Could you check a few things on this model? Use its own coordinates, in mm. Face numbers are marked on the shaded views. A direction names the side the tool comes from. Round coordinates to 2 decimals unless told otherwise and drop trailing zeros. Loops run counter-clockwise (first coordinate to the right, second up) from the corner with the lowest first, then second, coordinate; pieces in that order, holes last. Notation, with made-up numbers: M 19,-14.5 L 54,-14.5 A16 ccw 54,-6.5 Z; hole C 48,-10.75 d10. An arc over 180 degrees is marked long. Answer in a Markdown table with one row per item.
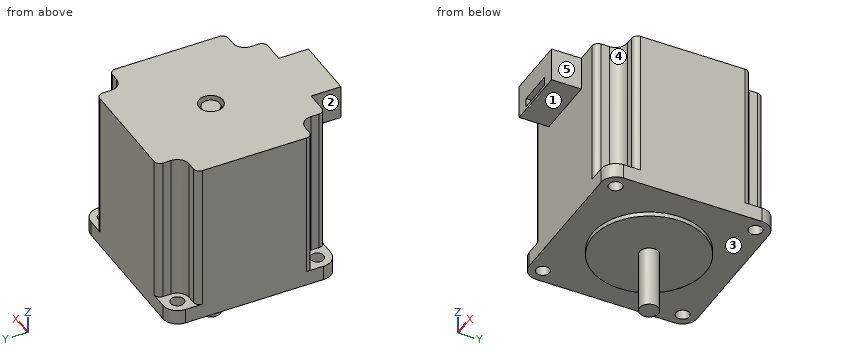
```python
from build123d import *

# Parameters (mm, degrees)
SKETCH_1_W          = 56.5
SKETCH_1_H          = 56.5
EXTRUDE_1_DEPTH     = 55
FILLET_1_R          = 5
SKETCH_2_W          = 27.937414654
SKETCH_2_H          = 17.525111135
CUT_EXTRUDE_1_DEPTH = 50
FILLET_2_R          = 4
FILLET_3_R          = 2
SKETCH_3_R          = 19
EXTRUDE_2_DEPTH     = 1.5
SKETCH_4_R          = 4
CUT_EXTRUDE_2_DEPTH = 3
SKETCH_5_R          = 3
EXTRUDE_3_DEPTH     = 2
SKETCH_6_R          = 3.175
EXTRUDE_4_DEPTH     = 21
SKETCH_7_R          = 2.25
CUT_EXTRUDE_3_DEPTH = 21
SKETCH_8_W          = 21
SKETCH_8_H          = 11.5
EXTRUDE_5_DEPTH     = 10
SKETCH_9_W          = 12
SKETCH_9_H          = 3
CUT_EXTRUDE_4_DEPTH = 5


with BuildPart() as part:
    # 草图1 → 凸台-拉伸1 (new body)
    with BuildSketch(Plane.XY):
        with Locations((28.25, 28.25)):
            Rectangle(SKETCH_1_W, SKETCH_1_H)
    extrude(amount=EXTRUDE_1_DEPTH)

    # 圆角1
    fillet_1_edges = [part.edges().sort_by_distance(p)[0] for p in [
        (0, 56.5, 27.5),
        (56.5, 56.5, 27.5),
        (56.5, 0, 27.5),
        (0, 0, 27.5),
    ]]
    fillet(fillet_1_edges, radius=FILLET_1_R)

    # 草图2 → 切除-拉伸1 (cut)
    with BuildSketch(Plane.XY.offset(55)):
        with Locations((-5.218707327, 56.512555568)):
            Rectangle(SKETCH_2_W, SKETCH_2_H)
        with Locations((61.718707327, 56.512555568)):
            Rectangle(SKETCH_2_W, SKETCH_2_H)
        with Locations((61.718707327, -0.012555568)):
            Rectangle(SKETCH_2_W, SKETCH_2_H)
        with Locations((-5.218707327, -0.012555568)):
            Rectangle(SKETCH_2_W, SKETCH_2_H)
    extrude(amount=-CUT_EXTRUDE_1_DEPTH, mode=Mode.SUBTRACT)

    # 圆角2
    fillet_2_edges = [part.edges().sort_by_distance(p)[0] for p in [
        (8.75, 8.75, 30),
        (8.75, 47.75, 30),
        (47.75, 47.75, 30),
        (47.75, 8.75, 30),
    ]]
    fillet(fillet_2_edges, radius=FILLET_2_R)

    # 圆角3
    fillet_3_edges = [part.edges().sort_by_distance(p)[0] for p in [
        (0, 8.75, 30),
        (8.75, 0, 30),
        (8.75, 56.5, 30),
        (0, 47.75, 30),
        (56.5, 47.75, 30),
        (47.75, 56.5, 30),
        (47.75, 0, 30),
        (56.5, 8.75, 30),
    ]]
    fillet(fillet_3_edges, radius=FILLET_3_R)

    # 草图3 → 凸台-拉伸2 (add)
    with BuildSketch(Plane(origin=(0, 0, 0), x_dir=(-1, 0, 0), z_dir=(0, 0, -1))):
        with Locations((-28.25, 28.25)):
            Circle(SKETCH_3_R)
    extrude(amount=EXTRUDE_2_DEPTH)

    # 草图4 → 切除-拉伸2 (cut)
    with BuildSketch(Plane.XY.offset(55)):
        with Locations((28.25, 28.25)):
            Circle(SKETCH_4_R)
    extrude(amount=-CUT_EXTRUDE_2_DEPTH, mode=Mode.SUBTRACT)

    # 草图5 → 凸台-拉伸3 (add)
    with BuildSketch(Plane.XY.offset(52)):
        with Locations((28.25, 28.25)):
            Circle(SKETCH_5_R)
    extrude(amount=EXTRUDE_3_DEPTH)

    # 草图6 → 凸台-拉伸4 (add)
    with BuildSketch(Plane(origin=(0, 0, -1.5), x_dir=(-1, 0, 0), z_dir=(0, 0, -1))):
        with Locations(Location((-28.25, 28.25, 0), (0, 0, 180))):
            Circle(SKETCH_6_R)
    extrude(amount=EXTRUDE_4_DEPTH)

    # 草图7 → 切除-拉伸3 (cut)
    with BuildSketch(Plane(origin=(0, 0, 0), x_dir=(-1, 0, 0), z_dir=(0, 0, -1))):
        with Locations((-51.8, 4.75)):
            Circle(SKETCH_7_R)
        with Locations((-4.7, 4.75)):
            Circle(SKETCH_7_R)
        with Locations((-4.7, 51.75)):
            Circle(SKETCH_7_R)
        with Locations((-51.8, 51.75)):
            Circle(SKETCH_7_R)
    extrude(amount=-CUT_EXTRUDE_3_DEPTH, mode=Mode.SUBTRACT)

    # 草图8 → 凸台-拉伸5 (add)
    with BuildSketch(Plane.XZ):
        with Locations((28.25, 49.25)):
            Rectangle(SKETCH_8_W, SKETCH_8_H)
    extrude(amount=EXTRUDE_5_DEPTH)

    # 草图9 → 切除-拉伸4 (cut)
    with BuildSketch(Plane.XZ.offset(10)):
        with Locations((28.25, 46)):
            Rectangle(SKETCH_9_W, SKETCH_9_H)
    extrude(amount=-CUT_EXTRUDE_4_DEPTH, mode=Mode.SUBTRACT)


solid = part.part
```
1) I need wall thicknesses on line 1 (Y direction, x = 4.7, z = 3.45); line 2 (Y direction, x = 51, z = 2); line 3 (Z direction, x = 6, y = 9.5). Which ranges of each line are inside material? Lowest first, please.
Computed:
| item | result |
|---|---|
| line 1 | y = 0.01 to 2.5, 7 to 49.5, 54 to 56.49 |
| line 2 | y = 0 to 2.65, 6.85 to 49.65, 53.85 to 56.5 |
| line 3 | z = 0 to 55 |
2) I want a section at B-B, the plane y = 28.25. Please give me the cut outline in (x, z) (3 decimals), plus the area to 3 significant figures.
Computed:
| item | result |
|---|---|
| outline | M 0,0 L 9.25,0 L 9.25,-1.5 L 25.075,-1.5 L 25.075,-22.5 L 31.425,-22.5 L 31.425,-1.5 L 47.25,-1.5 L 47.25,0 L 56.5,0 L 56.5,55 L 32.25,55 L 32.25,52 L 31.25,52 L 31.25,54 L 25.25,54 L 25.25,52 L 24.25,52 L 24.25,55 L 0,55 Z |
| area | 3,290 mm² |
3) I want a section at C-C, the plane x = 28.25. Please give me the cut outline in (y, z) (3 decimals).
Computed:
| item | result |
|---|---|
| outline | M -10,43.5 L 0,43.5 L 0,0 L 9.25,0 L 9.25,-1.5 L 25.075,-1.5 L 25.075,-22.5 L 31.425,-22.5 L 31.425,-1.5 L 47.25,-1.5 L 47.25,0 L 56.5,0 L 56.5,55 L 32.25,55 L 32.25,52 L 31.25,52 L 31.25,54 L 25.25,54 L 25.25,52 L 24.25,52 L 24.25,55 L -10,55 L -10,47.5 L -5,47.5 L -5,44.5 L -10,44.5 Z |
4) Will these pins go through, and if not, where does the flat tip stop? P1, Ø5, axis at x = 22.5, y = 24, coming from the -Z side; P2, Ø5, axis at y = -6, z = 51.5, coming from the -X side; P3, Ø2, axis at x = 53.5, z = 30, coming from the -Y side; P4, Ø2.5, axis at x = 4.7, y = 4.75, coming from the +Z side.
Computed:
| item | result |
|---|---|
| P1 | stops at z = -1.5 |
| P2 | stops at x = 17.75 |
| P3 | stops at y = 8.75 |
| P4 | passes through |
5) I want a section at A-A, the plane z = 50. Please give me the cut outline in (x, y).
Computed:
| item | result |
|---|---|
| outline | M 0,10.75 A2 ccw 2,8.75 L 4.75,8.75 A4 cw 8.75,4.75 L 8.75,2 A2 ccw 10.75,0 L 17.75,0 L 17.75,-10 L 38.75,-10 L 38.75,0 L 45.75,0 A2 ccw 47.75,2 L 47.75,4.75 A4 cw 51.75,8.75 L 54.5,8.75 A2 ccw 56.5,10.75 L 56.5,45.75 A2 ccw 54.5,47.75 L 51.75,47.75 A4 cw 47.75,51.75 L 47.75,54.5 A2 ccw 45.75,56.5 L 10.75,56.5 A2 ccw 8.75,54.5 L 8.75,51.75 A4 cw 4.75,47.75 L 2,47.75 A2 ccw 0,45.75 Z |
6) I want a section at D-D, the plane z = 27.5. Please give me the cut outline in (x, y).
Computed:
| item | result |
|---|---|
| outline | M 0,10.75 A2 ccw 2,8.75 L 4.75,8.75 A4 cw 8.75,4.75 L 8.75,2 A2 ccw 10.75,0 L 45.75,0 A2 ccw 47.75,2 L 47.75,4.75 A4 cw 51.75,8.75 L 54.5,8.75 A2 ccw 56.5,10.75 L 56.5,45.75 A2 ccw 54.5,47.75 L 51.75,47.75 A4 cw 47.75,51.75 L 47.75,54.5 A2 ccw 45.75,56.5 L 10.75,56.5 A2 ccw 8.75,54.5 L 8.75,51.75 A4 cw 4.75,47.75 L 2,47.75 A2 ccw 0,45.75 Z |
7) Which directions (+Z, -Z, +X, -X, +Y, -Y) give clear straight access to the entire face, cutting with the end or side of a thin tool? Please do the marked faces 1, 2, 3, 4 and 5.
Computed:
| item | result |
|---|---|
| face 1 | -Z, +X, -X, -Y |
| face 2 | +Z, -Z, -X, -Y |
| face 3 | -Z |
| face 4 | +Z, +X, -Y |
| face 5 | +Z, -Z, +X, -Y |
